```python
from build123d import *

# Parameters (mm, degrees)
EXTRUDE_1_DEPTH = 120
EXTRUDE_2_REACH = 151.666
EXTRUDE_3_DEPTH = 10


with BuildPart() as part:
    # 草圖1 → 填料-伸長1 (new body)
    with BuildSketch(Plane(origin=(0, 0, 0), x_dir=(0, 0, -1), z_dir=(1, 0, 0))):
        Polygon((-40, 0), (0, 0), (0, 70), (10, 70), (10, -10), (-40, -10), align=None)
    extrude(amount=EXTRUDE_1_DEPTH)

    # 草圖2 → 填料-伸長2 (add, up to next)
    with BuildSketch(Plane(origin=(0, 70, 0), x_dir=(1, 0, 0), z_dir=(0, 1, 0)), mode=Mode.PRIVATE) as extrude_2_sk1:
        Polygon((120, 0), (102.834521938, -24.603787572), (94.633259414, -18.881961552), (107.806755398, 0), align=None)
    extrude_2_tool1 = extrude(extrude_2_sk1.sketch, amount=-EXTRUDE_2_REACH, mode=Mode.PRIVATE) - part.part
    add(extrude_2_tool1.solids().sort_by_distance((106.542259, 70, 10.934177))[0])

    # 草圖3 → 填料-伸長3 (add)
    with BuildSketch(Plane(origin=(10, 0, 0), x_dir=(0, 0, -1), z_dir=(1, 0, 0))):
        Polygon((0, 70), (0, 0), (-40, 0), align=None)
    extrude(amount=EXTRUDE_3_DEPTH)


solid = part.part
```
Geometry: final body of the model. Coordinates: model frame, mm. A direction names the side the tool comes from. Round coordinates to 2 decimals unless told otherwise and drop trailing zeros. Write each loop counter-clockwise with the first axis right and the second up, starting at its lowest first coordinate (ties: lowest second). Pieces come first, ordered by that corner, then holes.
Item 1: Section query C-C (x = 29.5). Return loops of the section in (y, z), plus the area to 3 significant figures.
Item 2: Set-up query: faces 4 (the face through (111.537, 35.49, 12.13)), 5 (the face through (5, 0, 20)), 6 (the face through (20, 20, 11)). Return all of +Z, -Z, +X, -X, +Y, -Y with unobstructed straight access to the full face (end or side cutting, diameter ignored); none if empty.
Item 3: Section query D-D (y = 25). Return loops of the section in (x, z).
Item 4: Pin query (flat end, axial travel): P1, Ø3, axis at x = 4, z = 18.5, coming from the +Y side; P2, Ø8, axis at x = 17.5, z = 22, coming from the +Y side; P3, Ø1.5, axis at x = 81, y = 29.5, coming from the +Z side. Return the tip coordinate at first contact, or that it passes through.
Item 5: Mould query, pull axis Z, two halves, no side actions, for faces 1 (the face through (5, 35, 0)), 2 (the face through (59, -10, 15)), 3 (the face through (101.13, 35.49, 9.57)). Classes: +Z half, -Z half, draft (parallel to the pull), parting line (faces both ways), or undercut.
Item 6: Material intervals for L1, parallel to Y at x = 55, z = 30.5; L2, parallel to X at y = 53, z = 6, sorted ascending.
Item 7: Section query A-A (z = 29). Return loops of the section in (x, y).
Item 8: Section query B-B (y = 7). Return loops of the section in (x, z), plus the area to 3 significant figures.
Completed:
1. outline: (-10, -10) - (70, -10) - (70, 0) - (0, 0) - (0, 40) - (-10, 40) - close
1. area: 1,200 mm2
2. face 4: +Z, +X, +Y
2. face 5: +Z, -X, +Y
2. face 6: +Z, +Y
3. outline: (0, -10) - (120, -10) - (120, 0) - (102.83, 24.6) - (94.63, 18.88) - (107.81, 0) - (20, 0) - (20, 25.71) - (10, 25.71) - (10, 0) - (0, 0) - close
4. P1: stops at y = 0
4. P2: stops at y = 38.5
4. P3: stops at z = 0
5. face 1: +Z half
5. face 2: draft
5. face 3: undercut
6. L1: y = -10 to 0
6. L2: x = 10 to 20, 103.62 to 115.81
7. outline: (0, -10) - (120, -10) - (120, 0) - (20, 0) - (20, 19.25) - (10, 19.25) - (10, 0) - (0, 0) - close
8. outline: (0, -10) - (120, -10) - (120, 0) - (102.83, 24.6) - (94.63, 18.88) - (107.81, 0) - (20, 0) - (20, 36) - (10, 36) - (10, 0) - (0, 0) - close
8. area: 1,830 mm2
